The listing builds one solid part. Answer for the finished solid, in the listing's coordinates (mm). A direction names the side the tool comes from. Coordinates: 2 decimals unless noted, no trailing zeros. Write each loop counter-clockwise with the first axis right and the second up, starting at its lowest first coordinate (ties: lowest second). Pieces come first, ordered by that corner, then holes. Notation, with made-up numbers: M 21.25,-26 L 61.25,-26 A11 cw 61.25,-18 Z; hole C 19,-7 d4. An arc over 180 degrees is marked long. Answer as a JSON object with one key per item and string values. Group by question number.
from build123d import *

# Parameters (mm, degrees)
CROQUIS1_W              = 33
CROQUIS1_H              = 33
SALIENTE_EXTRUIR1_DEPTH = 6.6
CROQUIS2_W              = 29
CROQUIS2_H              = 29
CORTAR_EXTRUIR1_DEPTH   = 5
CROQUIS3_R              = 12
CORTAR_EXTRUIR2_DEPTH   = 5


with BuildPart() as part:
    # Croquis1 → Saliente-Extruir1 (new body)
    with BuildSketch(Plane(origin=(0, 0, 0), x_dir=(1, 0, 0), z_dir=(0, 1, 0))):
        Rectangle(CROQUIS1_W, CROQUIS1_H)
    extrude(amount=SALIENTE_EXTRUIR1_DEPTH)

    # Croquis2 → Cortar-Extruir1 (cut)
    with BuildSketch(Plane(origin=(0, 6.6, 0), x_dir=(1, 0, 0), z_dir=(0, 1, 0))):
        Rectangle(CROQUIS2_W, CROQUIS2_H)
    extrude(amount=-CORTAR_EXTRUIR1_DEPTH, mode=Mode.SUBTRACT)

    # Croquis3 → Cortar-Extruir2 (cut)
    with BuildSketch(Plane(origin=(0, 1.6, 0), x_dir=(1, 0, 0), z_dir=(0, 1, 0))):
        with Locations(Location((0, 0, 0), (0, 0, 270))):
            Circle(CROQUIS3_R)
    extrude(amount=-CORTAR_EXTRUIR2_DEPTH, mode=Mode.SUBTRACT)


solid = part.part
Item 1: A tool of negligible diameter and unlimited length cuts with its end or side. For faces 1 (the face through (-14.5, 4, 0)), 2 (the face through (16.5, 3, 0)), from which of +Z, -Z, +X, -X, +Y, -Y can it reach the whole face along a straight path? Write none if from no direction.
Item 2: Consider L1, parallel to X at y = 1.1, z = 0; L2, parallel to X at y = 5, z = -13. Determine where each line is inside the solid, lowest interval first. Write a range as from..to.
Item 3: A cutting plane is placed at D-D, the plane x = -13. Write down the section's boundary in (y, z).
Item 4: A cutting plane is placed at C-C, the plane y = 5.5. Write down the section's boundary in (x, z), and give its area (3 significant figures).
Item 5: For a pull along X with two mould halves and no side action, classify faces 3 (the face through (3.604, 0.811, 11.446)), 4 (the face through (-16.5, 3, 0)), 5 (the face through (-15, 6.6, 0)) as +X half, -X half, draft (parallel to the pull), parting line (faces both ways), or undercut.
Item 6: A cutting plane is placed at B-B, the plane x = 0. Write down the section's boundary in (y, z).
Item 7: A cutting plane is placed at A-A, the plane z = 0. Write down the section's boundary in (x, y), and give its area (3 significant figures).
Item 8: A flat-ended cylindrical pin translates along its axis: pin 1 Ø10 at (x, z) = (-8, -9) entering from +Y. Find the tip coordinate at first contact, or state that the pin passes through.
Answer:
{
 "1": {"face 1": "+Y", "face 2": "+Z, -Z, +X, +Y, -Y"},
 "2": {"L1": "-16.5..-12, 12..16.5", "L2": "-16.5..-14.5, 14.5..16.5"},
 "3": {"outline": "M 0,-16.5 L 6.6,-16.5 L 6.6,-14.5 L 1.6,-14.5 L 1.6,14.5 L 6.6,14.5 L 6.6,16.5 L 0,16.5 Z"},
 "4": {"outline": "M -16.5,-16.5 L 16.5,-16.5 L 16.5,16.5 L -16.5,16.5 Z; hole M -14.5,-14.5 L 14.5,-14.5 L 14.5,14.5 L -14.5,14.5 Z", "area": "248 mm2"},
 "5": {"face 3": "undercut", "face 4": "-X half", "face 5": "draft"},
 "6": {"outline": "M 0,-16.5 L 6.6,-16.5 L 6.6,-14.5 L 1.6,-14.5 L 1.6,-12 L 0,-12 Z; M 0,12 L 1.6,12 L 1.6,14.5 L 6.6,14.5 L 6.6,16.5 L 0,16.5 Z"},
 "7": {"outline": "M -16.5,0 L -12,0 L -12,1.6 L -14.5,1.6 L -14.5,6.6 L -16.5,6.6 Z; M 12,0 L 16.5,0 L 16.5,6.6 L 14.5,6.6 L 14.5,1.6 L 12,1.6 Z", "area": "34.4 mm2"},
 "8": {"pin 1": "y = 1.6"}
}
